Source: CAD feature listing. Evaluate the final solid. Frame: model axes, mm. A direction names the side the tool comes from. Give positions to 0.01 mm unless a question says otherwise; leave off trailing zeros. Write each loop counter-clockwise with the first axis right and the second up, starting at its lowest first coordinate (ties: lowest second). Pieces come first, ordered by that corner, then holes. Notation, with made-up numbers: (69, 6.5) -> (85, 6.5) arc R4 cw to (85, 12.5) -> close; hole circle Ø7 at (88, -2). An arc over 180 degrees is marked (long way). Write item = value, one per line.
from build123d import *

# Parameters (mm, degrees)
F0_W     = 152.4
F0_H     = 50.8
F0_W_2   = 139.7
F0_H_2   = 38.1
F1_DEPTH = 12.7
F2_W     = 27.94
F2_H     = 69.85
F2_W_2   = 8.89
F2_H_2   = 57.15
F3_DEPTH = 12.7
F4_R     = 2.54
F6_DEPTH = 12.701


with BuildPart() as f1:
    # F0 (on Top) → F1 (new body)
    with BuildSketch(Plane.XY):
        Rectangle(F0_W, F0_H)
        Rectangle(F0_W_2, F0_H_2, mode=Mode.SUBTRACT)
    extrude(amount=F1_DEPTH)

    # F2 (on Top) → F3 (join)
    with BuildSketch(Plane.XY):
        with Locations((-83.82, -3.175)):
            Rectangle(F2_W, F2_H)
        with Locations((-80.645, -3.175)):
            Rectangle(F2_W_2, F2_H_2, mode=Mode.SUBTRACT)
    extrude(amount=F3_DEPTH)

    # F4
    f4_edges = [f1.edges().sort_by_distance(p)[0] for p in [
        (-69.85, 19.05, 6.35),
        (69.85, 19.05, 6.35),
        (69.85, -19.05, 6.35),
        (-69.85, -19.05, 6.35),
        (-69.85, 25.4, 6.35),
        (76.2, 25.4, 6.35),
        (76.2, -25.4, 6.35),
        (-69.85, -25.4, 6.35),
        (-69.85, 31.75, 6.35),
        (-69.85, -38.1, 6.35),
    ]]
    fillet(f4_edges, radius=F4_R)

    # F5 (on face) → F6 (cut, through all)
    with BuildSketch(Plane(origin=(0, 0, 0), x_dir=(1, 0, 0), z_dir=(0, 0, -1))):
        Polygon((-97.79, -31.75), (-85.09, -31.75), (-85.09, -25.4), (-85.09, 31.75), (-85.09, 38.1), (-97.79, 38.1), align=None)
    extrude(amount=-F6_DEPTH, mode=Mode.SUBTRACT)


solid = f1.part
1) Cut plane C-C (z = 4.5). Return the cut outline in (x, y).
Computed:
outline = (-85.09, -38.1) -> (-72.39, -38.1) arc R2.54 ccw to (-69.85, -35.56) -> (-69.85, -27.94) arc R2.54 cw to (-67.31, -25.4) -> (73.66, -25.4) arc R2.54 ccw to (76.2, -22.86) -> (76.2, 22.86) arc R2.54 ccw to (73.66, 25.4) -> (-67.31, 25.4) arc R2.54 cw to (-69.85, 27.94) -> (-69.85, 29.21) arc R2.54 ccw to (-72.39, 31.75) -> (-85.09, 31.75) -> (-85.09, 25.4) -> (-76.2, 25.4) -> (-76.2, -31.75) -> (-85.09, -31.75) -> close; hole (-69.85, -16.51) arc R2.54 ccw to (-67.31, -19.05) -> (67.31, -19.05) arc R2.54 ccw to (69.85, -16.51) -> (69.85, 16.51) arc R2.54 ccw to (67.31, 19.05) -> (-67.31, 19.05) arc R2.54 ccw to (-69.85, 16.51) -> close
2) Cut plane A-A (y = 8.5). Return the cut outline in (x, z).
Computed:
outline = (-76.2, 0) -> (-69.85, 0) -> (-69.85, 12.7) -> (-76.2, 12.7) -> close; (69.85, 0) -> (76.2, 0) -> (76.2, 12.7) -> (69.85, 12.7) -> close
3) Contact query for flat-ended pins moving along their axis: pin 1 (6.5 mm diameter, centred on x = 6.5, z = 6, fed in from -Y); pin 2 (4 mm diameter, centred on y = -25, z = 8, fed in from +X); pin 3 (4 mm diameter, centred on x = -49.5, z = 7.5, fed in from +Y). Output: stop coordinate, or through.
Computed:
pin_1 = -25.4
pin_2 = 76.2
pin_3 = 25.4
4) Access query for faces 1 (the flat face through (2, -25.4, 6)), 2 (the flat face through (-1, -19.05, 6)), 3 (the flat face through (-81, 25.4, 6)). Directions: +Z, -Z, +X, -X, +Y, -Y. A direction counts if a zero-diameter tool reaches every point of the face in a straight line with its end or side. Return the directions, or none.
Computed:
face_1 = +Z, -Z, +X, -Y
face_2 = +Z, -Z
face_3 = +Z, -Z, -X
5) Material intervals for L1, parallel to X at y = 16, z = 3.75; L2, parallel to Y at x = 2.5, z = 4.25; L3, parallel to X at y = -17.5, z = 7.75, sorted ascending.
Computed:
L1 = -76.2 to -69.85, 69.85 to 76.2
L2 = -25.4 to -19.05, 19.05 to 25.4
L3 = -76.2 to -69.65, 69.65 to 76.2
6) Draft query along Y for faces 4 (the flat face through (-11, -21, 0)), 5 (the flat face through (-79, -38.1, 6)), 6 (the flat face through (-69.85, 0, 6)). Return one class per face: pulls with the +Y half, pulls with the -Y half, needs draft (parallel to the pull), parting line crosses it, or undercut.
Computed:
face_4 = needs draft
face_5 = pulls with the -Y half
face_6 = undercut
7) Cut plane B-B (x = -56). Return the cut outline in (y, z).
Computed:
outline = (-25.4, 0) -> (-19.05, 0) -> (-19.05, 12.7) -> (-25.4, 12.7) -> close; (19.05, 0) -> (25.4, 0) -> (25.4, 12.7) -> (19.05, 12.7) -> close
